from build123d import *

# Parameters (mm, degrees)
F0_R      = 3.325
F1_DEPTH  = 50
F2_R      = 5
F2_R_2    = 3.325
F3_DEPTH  = 2.85
F4_R      = 3.2
F5_DEPTH  = 7.9
F6_R      = 1
F7_DEPTH  = 55
F8_R      = 2.05
F9_DEPTH  = 6.9
F10_R     = 2.5
F10_R_2   = 1.75
F11_DEPTH = 4


with BuildPart() as f1:
    # F0 (on Top) → F1 (new body)
    with BuildSketch(Plane.XY):
        Circle(F0_R)
    extrude(amount=F1_DEPTH)

    # F2 (on face) → F3 (join)
    with BuildSketch(Plane.XY):
        Circle(F2_R)
        Circle(F2_R_2, mode=Mode.SUBTRACT)
        Circle(F2_R)
    extrude(amount=-F3_DEPTH)

    # F4 (on face) → F5 (join)
    with BuildSketch(Plane(origin=(0, 0, -2.85), x_dir=(1, 0, 0), z_dir=(0, 0, -1))):
        Circle(F4_R)
    extrude(amount=F5_DEPTH)

    # F6 (on face) → F7 (cut)
    with BuildSketch(Plane.XY.offset(50)):
        Circle(F6_R)
    extrude(amount=-F7_DEPTH, mode=Mode.SUBTRACT)

    # F8 (on face) → F9 (cut)
    with BuildSketch(Plane(origin=(0, 0, -10.75), x_dir=(1, 0, 0), z_dir=(0, 0, -1))):
        Circle(F8_R)
    extrude(amount=-F9_DEPTH, mode=Mode.SUBTRACT)

    # F10 (on Front) → F11 (cut, symmetric)
    with BuildSketch(Plane.XZ):
        with Locations((-3, 50)):
            Circle(F10_R)
        with Locations((2, 50)):
            Circle(F10_R_2)
    extrude(amount=F11_DEPTH, both=True, mode=Mode.SUBTRACT)


solid = f1.part
Work out the finished part from the listing and answer in its coordinate system (mm). A direction names the side the tool comes from. Give positions to 0.01 mm unless a question says otherwise; leave off trailing zeros. Loops run counter-clockwise (first coordinate to the right, second up) from the corner with the lowest first, then second, coordinate; pieces in that order, holes last. Notation, with made-up numbers: (23.5, 72.5) -> (29.5, 72.5) arc R24 cw to (29.5, 100.5) -> close; hole circle Ø6 at (-26.75, 66.25). An arc over 180 degrees is marked (long way). Use a Markdown table: item, result. Add a question column.
1) The part is cut by section B-B, the plane y = 1.5. Determine the outline of the cut face in (x, z), plus the area to 3 significant figures.
2) For a pull along X with two mould halves and no side action, classify faces 1 (the cylindrical face through (-0.267, -2.033, -7.348)), 2 (the cylindrical face through (-1.08, -4.88, -1.41)), 3 (the flat face through (-1.2, -3.3, 0)) as +X half, -X half, draft (parallel to the pull), parting line (faces both ways), or undercut.
3) The part is cut by section A-A, the plane z = 11.5. Determine the outline of the cut face in (x, y) (3 decimals), plus the area to 3 significant figures.
4) Which of the six approach directions +Z, -Z, +X, -X, +Y, -Y give full straight-line access (tool end or side, diameter ignored) to faces 4 (the flat face through (1, -3.3, -2.85)), 5 (the cylindrical face through (1.36, -0.05, 48.37)), 6 (the cylindrical face through (1.53, -2.95, 24.65))?
5) Consider line 1 along X through (y, z) = (0, -9); line 2 along Y through (x, z) = (0, 31) (3 decimals). Determine where each line is inside the solid, lowest interval first.
6) Each of these flat-tipped pins is pushed along its axis until it touches: P1, Ø3, axis at x = 2, y = -2.5, coming from the +Z side; P2, Ø4, axis at y = 3, z = 38, coming from the +X side; P3, Ø3.5, axis at x = 0, y = 0, coming from the -Z side; P4, Ø4.5, axis at x = -1, y = -0.5, coming from the -Z side. Where does it stop, or does it pass through?
Reported:
| question | item | result |
|---|---|---|
| 1 | outline | (-4.77, -2.85) -> (-2.83, -2.85) -> (-2.83, -10.75) -> (-1.4, -10.75) -> (-1.4, -3.85) -> (1.4, -3.85) -> (1.4, -10.75) -> (2.83, -10.75) -> (2.83, -2.85) -> (4.77, -2.85) -> (4.77, 0) -> (2.97, 0) -> (2.97, 48.54) arc R1.75 cw to (0.25, 50) -> (-0.5, 50) arc R2.5 cw to (-2.97, 47.5) -> (-2.97, 0) -> (-4.77, 0) -> close |
| 1 | area | 340 mm^2 |
| 2 | face 1 | undercut |
| 2 | face 2 | parting line |
| 2 | face 3 | draft |
| 3 | outline | circle Ø6.65 at (0, 0); hole circle Ø2 at (0, 0) |
| 3 | area | 31.6 mm^2 |
| 4 | face 4 | -Z |
| 4 | face 5 | +Z, +Y, -Y |
| 4 | face 6 | +Z |
| 5 | line 1 | x = -3.2 to -2.05, 2.05 to 3.2 |
| 5 | line 2 | y = -3.325 to -1, 1 to 3.325 |
| 6 | P1 | stops at z = 49.1 |
| 6 | P2 | stops at x = 3.17 |
| 6 | P3 | stops at z = -3.85 |
| 6 | P4 | stops at z = -10.75 |
